```python
from build123d import *

# Parameters (mm, degrees)
SKETCH1_W           = 78
SKETCH1_H           = 70
SKETCH1_W_2         = 48
SKETCH1_H_2         = 40
SKETCH1_W_3         = 5
SKETCH1_H_3         = 6.5
SKETCH1_R           = 1.5
BOSS_EXTRUDE2_DEPTH = 1
FILLET2_R           = 10
FILLET3_R           = 2


with BuildPart() as part:
    # Sketch1 → Boss-Extrude2 (new body)
    # profile 1 of 6: a face of its own
    with BuildSketch(Plane.XY):
        with Locations((-0.075399098, 4.950190099)):
            Rectangle(SKETCH1_W, SKETCH1_H)
        with Locations((-0.075399098, 4.950190099)):
            Rectangle(SKETCH1_W_2, SKETCH1_H_2, mode=Mode.SUBTRACT)
        with Locations((-29.575399098, -20.799809901)):
            Rectangle(SKETCH1_W_3, SKETCH1_H_3, mode=Mode.SUBTRACT)
        with Locations((-29.575399098, 30.700190099)):
            Rectangle(SKETCH1_W_3, SKETCH1_H_3, mode=Mode.SUBTRACT)
        with Locations((29.424600902, 30.700190099)):
            Rectangle(SKETCH1_W_3, SKETCH1_H_3, mode=Mode.SUBTRACT)
        with Locations((29.424600902, -20.799809901)):
            Rectangle(SKETCH1_W_3, SKETCH1_H_3, mode=Mode.SUBTRACT)
    # profile 2 of 6: a face of its own
    with BuildSketch(Plane.XY):
        with Locations((29.424600902, -20.799809901)):
            Rectangle(SKETCH1_W_3, SKETCH1_H_3)
        with Locations((29.424600902, -20.799809901)):
            Circle(SKETCH1_R, mode=Mode.SUBTRACT)
    # profile 3 of 6: a face of its own
    with BuildSketch(Plane.XY):
        with Locations((-29.575399098, -20.799809901)):
            Rectangle(SKETCH1_W_3, SKETCH1_H_3)
        with Locations((-29.575399098, -20.799809901)):
            Circle(SKETCH1_R, mode=Mode.SUBTRACT)
    # profile 4 of 6: a face of its own
    with BuildSketch(Plane.XY):
        with Locations((29.424600902, 30.700190099)):
            Rectangle(SKETCH1_W_3, SKETCH1_H_3)
        with Locations((29.424600902, 30.700190099)):
            Circle(SKETCH1_R, mode=Mode.SUBTRACT)
    # profile 5 of 6: a face of its own
    with BuildSketch(Plane.XY):
        Polygon((23.924600902, 24.950190099), (-24.075399098, 24.950190099), (-24.075399098, -15.049809901), (-10.075399098, -15.049809901), (-10.075399098, -7.049809901), (9.924600902, -7.049809901), (9.924600902, -15.049809901), (23.924600902, -15.049809901), align=None)
    # profile 6 of 6: a face of its own
    with BuildSketch(Plane.XY):
        with Locations((-29.575399098, 30.700190099)):
            Rectangle(SKETCH1_W_3, SKETCH1_H_3)
        with Locations((-29.575399098, 30.700190099)):
            Circle(SKETCH1_R, mode=Mode.SUBTRACT)
    extrude(amount=BOSS_EXTRUDE2_DEPTH)

    # Fillet2
    fillet2_edges = [part.edges().sort_by_distance(p)[0] for p in [
        (38.924600902, -30.049809901, 0.5),
        (-39.075399098, -30.049809901, 0.5),
        (-39.075399098, 39.950190099, 0.5),
        (38.924600902, 39.950190099, 0.5),
    ]]
    fillet(fillet2_edges, radius=FILLET2_R)

    # Fillet3
    fillet3_edges = [part.edges().sort_by_distance(p)[0] for p in [
        (9.924600902, -15.049809901, 0.5),
        (9.924600902, -7.049809901, 0.5),
        (-10.075399098, -7.049809901, 0.5),
        (-10.075399098, -15.049809901, 0.5),
    ]]
    fillet(fillet3_edges, radius=FILLET3_R)


solid = part.part
```
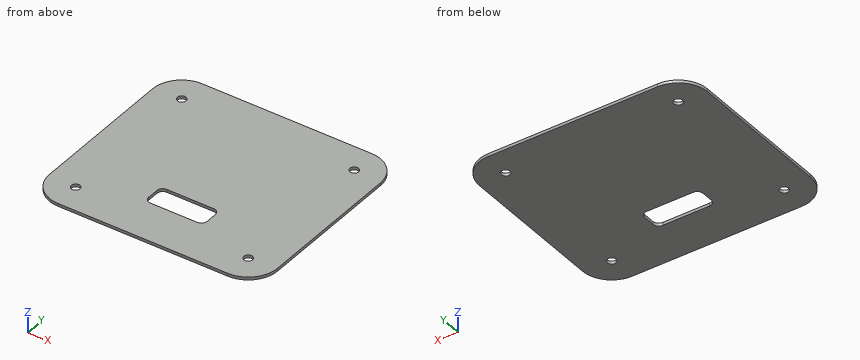
For this review, take the finished solid that the model builds, in its own axes (mm). Give positions to 0.01 mm unless a question says otherwise; leave off trailing zeros. Loops run counter-clockwise (first coordinate to the right, second up) from the corner with the lowest first, then second, coordinate; pieces in that order, holes last. Notation, with made-up numbers: M 78,-18 L 123,-18 A26 cw 123,8 Z; hole C 70,-26.75 d6. An arc over 180 degrees is marked long. One line per item, written item: value. Start each with the question number.
Q1. Add section B-B (z = 0.85). Give the boundary of the cut face in (x, y).
Q2. Add section A-A (x = 5). Give the boundary of the cut face in (y, z).
Q3. For L1, parallel to X at y = -9, z = 0.35; L2, parallel to Y at x = 8, z = 0.5; L3, parallel to Y at x = -30.5, z = 0.75, list the stretches that pass through material, from the lowest coordinate up.
Q4. Add section C-C (x = -9). Give the boundary of the cut face in (y, z), and give its area (3 significant figures).
Q5. Add section D-D (x = -33). Give the boundary of the cut face in (y, z), and give its area (3 significant figures).
Reply:
1. outline: M -39.08,-20.05 A10 ccw -29.08,-30.05 L 28.92,-30.05 A10 ccw 38.92,-20.05 L 38.92,29.95 A10 ccw 28.92,39.95 L -29.08,39.95 A10 ccw -39.08,29.95 Z; hole C -29.58,-20.8 d3; hole C -29.58,30.7 d3; hole M -10.08,-13.05 A2 ccw -8.08,-15.05 L 7.92,-15.05 A2 ccw 9.92,-13.05 L 9.92,-9.05 A2 ccw 7.92,-7.05 L -8.08,-7.05 A2 ccw -10.08,-9.05 Z; hole C 29.42,-20.8 d3; hole C 29.42,30.7 d3
2. outline: M -30.05,0 L -15.05,0 L -15.05,1 L -30.05,1 Z; M -7.05,0 L 39.95,0 L 39.95,1 L -7.05,1 Z
3. L1: -39.08 to -10.07, 9.92 to 38.92
3. L2: -30.05 to -15.05, -7.05 to 39.95
3. L3: -29.95 to -21.98, -19.62 to 29.52, 31.88 to 39.85
4. outline: M -30.05,0 L -14.82,0 L -14.82,1 L -30.05,1 Z; M -7.28,0 L 39.95,0 L 39.95,1 L -7.28,1 Z
4. area: 62.5 mm²
5. outline: M -29.25,0 L 39.15,0 L 39.15,1 L -29.25,1 Z
5. area: 68.4 mm²
